Work out the finished part from the listing and answer in its coordinate system (mm). A direction names the side the tool comes from. Round coordinates to 2 decimals unless told otherwise and drop trailing zeros. Loops run counter-clockwise (first coordinate to the right, second up) from the corner with the lowest first, then second, coordinate; pieces in that order, holes last. Notation, with made-up numbers: (23.25, 29) - (72.25, 29) arc R8 ccw to (72.25, 41) - close; hole circle Ø8 at (11.5, -12.5). An arc over 180 degrees is marked (long way). Return JSON: item names as keys, results as strings.
from build123d import *


with BuildPart() as part:
    # Croquis1 → Revolución1 (revolve)
    with BuildSketch(Plane.XY, mode=Mode.PRIVATE) as revoluci_n1_sk:
        with BuildLine():
            Line((0, 250), (-15, 250))
            Line((-15, 250), (-15, 235))
            Line((-15, 235), (-18, 235))
            Line((-18, 235), (-18, 233.5))
            Line((-18, 233.5), (-15, 233.5))
            Line((-15, 233.5), (-15, 227.283149652))
            add(Edge.make_bspline(
                [(-15, 227.283149652), (-16.277986715, 219.305420885), (-19.489344326, 206.260916929), (-32.684348565, 194.323220301), (-38.547275622, 176.702280824), (-39.162662254, 152.86461741), (-33.561571476, 127.462649854), (-30.990721493, 94.977950046), (-48.241664637, 54.863367585), (-44.557007193, 17.989663347), (-35, 0)],
                knots=[0, 0, 0, 0, 0.105527687, 0.159807734, 0.221005565, 0.335010102, 0.459707985, 0.552192154, 0.743984647, 1, 1, 1, 1], degree=3))
            Line((-35, 0), (0, 0))
            Line((0, 0), (0, 250))
        make_face()
    revolve(revoluci_n1_sk.sketch.rotate(Axis((0, 0, 0), (0, 1, 0)), 270), axis=Axis((0, 0, 0), (0, 1, 0)))


solid = part.part
1) Find the intervals of material crossed by L1, parallel to Z at x = -0.5, y = 236; L2, parallel to Z at x = -6.5, y = 129.5; L3, parallel to X at y = 79.5, z = -30, in increasing order.
Verdict:
{"L1": "z = -14.99 to 14.99", "L2": "z = -33.86 to 33.86", "L3": "x = -22.72 to 22.72"}
2) Section A-A (y = 230.5) is taken. Give the vertices of the cut face in (x, z), and give its area (3 significant figures).
Verdict:
{"outline": "circle Ø30 at (0, 0)", "area": "707 mm2"}
3) Flat-ended cylindrical pins translate along their axes: pin 1 (5 mm diameter, centred on y = 141, z = -0.5, fed in from +X); pin 2 (5 mm diameter, centred on x = 8, y = 85.5, fed in from -Z); pin 3 (10 mm diameter, centred on y = 153.5, z = -16.5, fed in from -X). Find the tip coordinate at first contact, or state that the pin passes through.
Verdict:
{"pin 1": "stops at x = 36.79", "pin 2": "stops at z = -35.94", "pin 3": "stops at x = -36.36"}
4) Determine the mould class of faces 1 (the cylindrical face through (-0.66, 230.348, 14.985)), 2 (the flat face through (-15, 235, -4)), 3 (the cylindrical face through (-5.407, 234.24, -17.169)) for opening direction Y: pulls with the +Y half, pulls with the -Y half, needs draft (parallel to the pull), parting line crosses it, or undercut.
Verdict:
{"face 1": "undercut", "face 2": "pulls with the +Y half", "face 3": "needs draft"}
5) A tool of negligible diameter and unlimited length cuts with its end or side. For faces 4 (the cylindrical face through (-0.66, 242.395, 14.985)), 5 (the flat face through (0, 250, 0)), 6 (the flat face through (-15, 233.5, 4)), from which of +Z, -Z, +X, -X, +Y, -Y can it reach the whole face along a straight path? Write none if from no direction.
Verdict:
{"face 4": "+Y", "face 5": "+Z, -Z, +X, -X, +Y", "face 6": "none"}
